Could you check a few things on this model? Use its own coordinates, in mm. Face numbers are marked on the shaded views. A direction names the side the tool comes from. Coordinates: 2 decimals unless noted, no trailing zeros. Loops run counter-clockwise (first coordinate to the right, second up) from the corner with the lowest first, then second, coordinate; pieces in that order, holes last. Notation, with made-up numbers: (89.25, -33.75) -> (146.25, -33.75) arc R34 ccw to (146.25, -2.75) -> close; hole circle Ø11 at (-32, -22). An arc over 180 degrees is marked (long way). One line per question, with ' | ' between items.
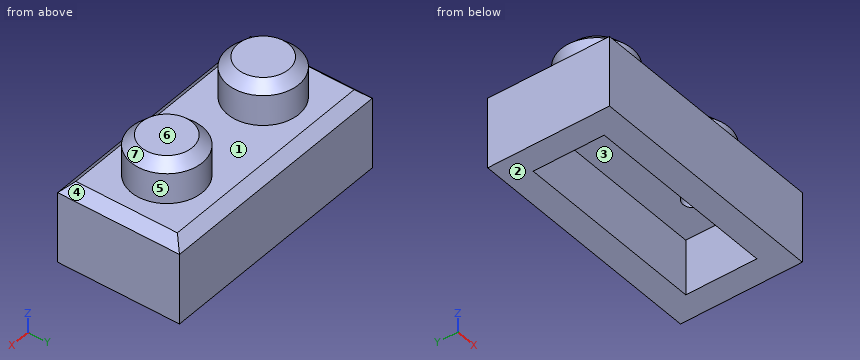
```python
from build123d import *

# Parameters (mm, degrees)
F0_W     = 76.2
F0_H     = 38.1
F1_DEPTH = 25.4
F2_R     = 11.1125
F3_DEPTH = 12.7
F4_T     = -7.9375
F5_SIZE2 = 3.175
F5_SIZE  = 3.175


with BuildPart() as f1:
    # F0 (on Top) → F1 (new body)
    with BuildSketch(Plane.XY):
        with Locations((38.1, 19.05)):
            Rectangle(F0_W, F0_H)
    extrude(amount=F1_DEPTH)

    # F2 (on face) → F3 (join)
    with BuildSketch(Plane.XY.offset(25.4)):
        with Locations((19.05, 19.05)):
            Circle(F2_R)
        with Locations((57.15, 19.05)):
            Circle(F2_R)
    extrude(amount=F3_DEPTH)

    # F4
    f4_openings = [f1.faces().sort_by_distance(p)[0] for p in [
        (38.1, 19.05, 0),
    ]]
    offset(amount=F4_T, openings=f4_openings, kind=Kind.INTERSECTION)

    # F5
    f5_edges = [f1.edges().sort_by_distance(p)[0] for p in [
        (7.9375, 19.05, 38.1),
        (46.0375, 19.05, 38.1),
        (38.1, 0, 25.4),
        (38.1, 38.1, 25.4),
        (0, 19.05, 25.4),
        (76.2, 19.05, 25.4),
    ]]
    chamfer(f5_edges, length=F5_SIZE, length2=F5_SIZE2)


solid = f1.part
```
Q1. Imagine slicing it at C-C on z = 15. Write out the boundary of the cut face in (x, y).
Values follow:
outline: (0, 0) -> (76.2, 0) -> (76.2, 38.1) -> (0, 38.1) -> close; hole (7.94, 7.94) -> (68.26, 7.94) -> (68.26, 30.16) -> (7.94, 30.16) -> close
Q2. For pin 1 (5 mm diameter, centred on y = 8.5, z = 25, fed in from +X) (3 decimals); pin 2 (7 mm diameter, centred on x = 19, y = 18, fed in from -Z); pin 3 (3 mm diameter, centred on x = 57.5, y = 17.5, fed in from -Z), each with a flat end and sliding along its axis, tell me the tip position at first contact or that it passes through.
Values follow:
pin 1: stops at x = 75.925 | pin 2: stops at z = 17.46 | pin 3: stops at z = 30.16
Q3. We'd pull the mould along X, two halves only. Please class the marked faces 4, 5, 6 and 7: released by +X, released by -X, zero draft, split by the parting line, or undercut.
Values follow:
face 4: released by +X | face 5: undercut | face 6: zero draft | face 7: undercut
Q4. Please list where these lines run through material, in increasing order: L1, parallel to X at y = 19, z = 27; L2, parallel to X at y = 19.05, z = 20.5 (3 decimals); L3, parallel to Y at x = 57, z = 22. Write a range as [from, to].
Values follow:
L1: x = [7.94, 15.88], [22.22, 30.16], [46.04, 53.98], [60.32, 68.26] | L2: x = [0, 15.875], [22.225, 53.975], [60.325, 76.2] | L3: y = [0, 15.88], [22.22, 38.1]
Q5. For the marked faces 1, 2 and 3, which set-ups out of +Z, -Z, +X, -X, +Y, -Y let a thin tool reach every point of the face, with its end or its side?
Values follow:
face 1: +Z | face 2: -Z, +X, -X, +Y, -Y | face 3: -Z
Q6. Imagine slicing it at A-A on z = 21. Write out the boundary of the cut face in (x, y) (3 decimals).
Values follow:
outline: (0, 0) -> (76.2, 0) -> (76.2, 38.1) -> (0, 38.1) -> close; hole circle Ø6.35 at (19.05, 19.05); hole circle Ø6.35 at (57.15, 19.05)
Q7. Imagine slicing it at B-B on x = 19.05. Write out the boundary of the cut face in (y, z) (1 decimal).
Values follow:
outline: (0, 0) -> (7.9, 0) -> (7.9, 17.5) -> (15.9, 17.5) -> (15.9, 30.2) -> (22.2, 30.2) -> (22.2, 17.5) -> (30.2, 17.5) -> (30.2, 0) -> (38.1, 0) -> (38.1, 22.2) -> (34.9, 25.4) -> (30.2, 25.4) -> (30.2, 34.9) -> (27, 38.1) -> (11.1, 38.1) -> (7.9, 34.9) -> (7.9, 25.4) -> (3.2, 25.4) -> (0, 22.2) -> close
